from build123d import *

# Parameters (mm, degrees)
SKETCH2_R          = 4.5
CUT_EXTRUDE1_DEPTH = 0.1
CUT_EXTRUDE2_DEPTH = 0.1
SKETCH4_W          = 0.3
SKETCH4_H          = 2.5
FILLET1_R          = 0.5


with BuildPart() as part:
    # Sketch1 → Revolve1 (revolve)
    with BuildSketch(Plane.XY, mode=Mode.PRIVATE) as revolve1_sk:
        with BuildLine():
            Line((5, 12.5), (0, 12.5))
            Line((0, 12.5), (0, 0))
            Line((0, 0), (4.827244523, 0))
            ThreePointArc((4.827244523, 0), (4.933458385, 0.471594976), (4.82617218, 0.942947155))
            ThreePointArc((4.82617218, 0.942947155), (4.777062056, 1.084088077), (4.760416667, 1.232599004))
            Line((4.760416667, 1.232599004), (4.760416667, 1.642400996))
            ThreePointArc((4.760416667, 1.642400996), (4.791064683, 1.842850794), (4.880208333, 2.024984899))
            ThreePointArc((4.880208333, 2.024984899), (4.969351983, 2.207119004), (5, 2.407568802))
            Line((5, 2.407568802), (5, 12.5))
        make_face()
    revolve(revolve1_sk.sketch.rotate(Axis((0, 12.5, 0), (0, -1, 0)), 270), axis=Axis((0, 12.5, 0), (0, -1, 0)))

    # Sketch2 → Cut-Extrude1 (cut)
    with BuildSketch(Plane(origin=(0, 12.5, 0), x_dir=(-1, 0, 0), z_dir=(0, 1, 0))):
        with Locations(Location((0, 0, 0), (0, 0, 270))):
            Circle(SKETCH2_R)
    extrude(amount=-CUT_EXTRUDE1_DEPTH, mode=Mode.SUBTRACT)

    # Sketch3 → Cut-Extrude2 (cut)
    with BuildSketch(Plane(origin=(0, 12.4, 0), x_dir=(-1, 0, 0), z_dir=(0, 1, 0))):
        Polygon((2.906036622, -3.256093686), (3.090537324, -3.081521376), (0.142645036, 0.03402539), (1.320649975, 3.989641976), (1.07721557, 4.062138116), (-0.10078937, 0.10652153), (-4.155587963, -0.860677244), (-4.096654259, -1.107745693), (-0.041855666, -0.14054692), align=None)
    extrude(amount=-CUT_EXTRUDE2_DEPTH, mode=Mode.SUBTRACT)

    # Sketch4 → Revolve2 (revolve)
    with BuildSketch(Plane(origin=(0, 0, 0), x_dir=(-1, 0, 0), z_dir=(0, 0, -1)), mode=Mode.PRIVATE) as revolve2_sk:
        with Locations((-2.65, -1.25)):
            Rectangle(SKETCH4_W, SKETCH4_H)
    revolve2 = revolve(revolve2_sk.sketch.rotate(Axis((2.5, -2.5, 0), (0, 1, 0)), 270), axis=Axis((2.5, -2.5, 0), (0, 1, 0)))

    # Fillet1
    fillet1_edges = [part.edges().sort_by_distance(p)[0] for p in [
        (0, 12.5, 5),
        (0, 0, 4.827244523),
    ]]
    fillet(fillet1_edges, radius=FILLET1_R - 0.0001)  # a hair under: the kernel refuses the full size

    # Simetría3: Revolve2 across plane
    add(revolve2.mirror(Plane(origin=(0, 0, 0), x_dir=(0, 0, 1), z_dir=(1, 0, 0))))


solid = part.part
Build history of the part. All positions in model axes, mm. Give positions to 0.01 mm unless a question says otherwise; leave off trailing zeros. Write each loop counter-clockwise with the first axis right and the second up, starting at its lowest first coordinate (ties: lowest second). Pieces come first, ordered by that corner, then holes. Notation, with made-up numbers: (51.5, -28.75) - (68.5, -28.75) arc R19 ccw to (68.5, 0.25) - close; hole circle Ø2 at (79, 23). An arc over 180 degrees is marked (long way). Use one line per item in the form item = value. Start each with the question number.
1. Probe line 1 (Y direction, x = -2.5, z = -0.75); line 2 (Z direction, x = -2.25, y = -1); line 3 (Z direction, x = -0.5, y = 0.75). List the from-to ranges inside material, lowest first. Write a range as [from, to].
2. Band-saw the part on A-A on y = -0.25. Write the cut outline in (x, z), plus the area to 3 significant figures.
3. Band-saw the part on B-B on y = 6.25. Write the cut outline in (x, z).
4. Drop flat-ended pins along their axis: pin 1 Ø2.5 at (x, z) = (-1, 0) entering from +Y; pin 2 Ø1 at (x, y) = (2, 4.5) entering from +Z; pin 3 Ø1 at (x, y) = (3.5, 11) entering from +Z. Give the stop position or say it passes through.
5. Two-plate mould, pull along Z, no slides. Class faces 1 (the face through (0, 0, 0)), 2 (the face through (0, 12.4, -1)), 3 (the face through (-4.647, 1.44, 1.032)): released by +Z, released by -Z, zero draft, split by the parting line, or undercut.
Conclusion:
q1.line_1 = [0, 12.4]
q1.line_2 = [-0.17, 0.17]
q1.line_3 = [-4.87, 4.87]
q2.outline = circle Ø0.6 at (-2.5, 0); circle Ø0.6 at (2.5, 0)
q2.area = 0.565 mm²
q3.outline = circle Ø10 at (0, 0)
q4.pin_1 = 12.4
q4.pin_2 = 4.77
q4.pin_3 = 4
q5.face_1 = zero draft
q5.face_2 = undercut
q5.face_3 = split by the parting line
